from build123d import *

# Parameters (mm, degrees)
BOSS_EXTRU_1_DEPTH = 5
CONG_1_R           = 3


with BuildPart() as part:
    # Esquisse1 → Boss.-Extru.1 (new body)
    with BuildSketch(Plane.XY):
        with BuildLine():
            Line((0, -5), (0, 0))
            Line((0, 0), (-15, 0))
            Line((-15, 0), (-21.92820323, -9.797958971))
            Line((-21.92820323, -9.797958971), (-26.010686135, -6.911207626))
            Line((-26.010686135, -6.911207626), (-28.89743748, -10.99369053))
            Line((-28.89743748, -10.99369053), (-24.814954576, -13.880441876))
            Line((-24.814954576, -13.880441876), (-26.835680518, -16.73817991))
            Line((-26.835680518, -16.73817991), (-24.386190775, -18.470230717))
            Line((-24.386190775, -18.470230717), (-23.751105479, -17.572084478))
            Line((-23.751105479, -17.572084478), (-21.873163342, -18.899990097))
            Line((-21.873163342, -18.899990097), (-22.508248639, -19.798136336))
            Line((-22.508248639, -19.798136336), (-18.670714708, -22.511682601))
            Line((-18.670714708, -22.511682601), (-20.402765515, -24.961172344))
            Line((-20.402765515, -24.961172344), (-24.240299446, -22.247626079))
            Line((-24.240299446, -22.247626079), (-24.875384742, -23.145772318))
            Line((-24.875384742, -23.145772318), (-26.753326878, -21.817866699))
            Line((-26.753326878, -21.817866699), (-26.118241582, -20.91972046))
            Line((-26.118241582, -20.91972046), (-28.567731325, -19.187669652))
            Line((-28.567731325, -19.187669652), (-30.588457267, -22.045407686))
            Line((-30.588457267, -22.045407686), (-34.670940172, -19.15865634))
            Line((-34.670940172, -19.15865634), (-37.557691518, -23.241139245))
            Line((-37.557691518, -23.241139245), (-33.475208613, -26.127890591))
            Line((-33.475208613, -26.127890591), (-36.361959959, -30.210373495))
            Line((-36.361959959, -30.210373495), (-40.444442863, -27.32362215))
            Line((-40.444442863, -27.32362215), (-43.331194209, -31.406105054))
            Line((-43.331194209, -31.406105054), (-39.248711304, -34.2928564))
            Line((-39.248711304, -34.2928564), (-41.269437246, -37.150594433))
            Line((-41.269437246, -37.150594433), (-38.819947503, -38.882645241))
            Line((-38.819947503, -38.882645241), (-38.184862207, -37.984499002))
            Line((-38.184862207, -37.984499002), (-36.306920071, -39.312404621))
            Line((-36.306920071, -39.312404621), (-36.942005367, -40.21055086))
            Line((-36.942005367, -40.21055086), (-33.104471437, -42.924097125))
            Line((-33.104471437, -42.924097125), (-34.836522244, -45.373586868))
            Line((-34.836522244, -45.373586868), (-38.674056175, -42.660040603))
            Line((-38.674056175, -42.660040603), (-39.309141471, -43.558186842))
            Line((-39.309141471, -43.558186842), (-41.187083607, -42.230281223))
            Line((-41.187083607, -42.230281223), (-40.551998311, -41.332134984))
            Line((-40.551998311, -41.332134984), (-43.001488054, -39.600084176))
            Line((-43.001488054, -39.600084176), (-45.022213996, -42.45782221))
            Line((-45.022213996, -42.45782221), (-49.104696901, -39.571070864))
            Line((-49.104696901, -39.571070864), (-51.991448246, -43.653553769))
            Line((-51.991448246, -43.653553769), (-47.908965342, -46.540305114))
            Line((-47.908965342, -46.540305114), (-50.795716687, -50.622788019))
            ThreePointArc((-50.795716687, -50.622788019), (-33.780137683, -59.08727806), (-15, -62))
            Line((-15, -62), (0, -62))
            Line((0, -62), (0, -57))
            Line((0, -57), (5, -57))
            Line((5, -57), (5, -52))
            Line((5, -52), (0, -52))
            Line((0, -52), (0, -48.5))
            Line((0, -48.5), (-3, -48.5))
            Line((-3, -48.5), (-3, -49.6))
            Line((-3, -49.6), (-5.3, -49.6))
            Line((-5.3, -49.6), (-5.3, -48.5))
            Line((-5.3, -48.5), (-10, -48.5))
            Line((-10, -48.5), (-10, -45.5))
            Line((-10, -45.5), (-5.3, -45.5))
            Line((-5.3, -45.5), (-5.3, -44.4))
            Line((-5.3, -44.4), (-3, -44.4))
            Line((-3, -44.4), (-3, -45.5))
            Line((-3, -45.5), (0, -45.5))
            Line((0, -45.5), (0, -42))
            Line((0, -42), (5, -42))
            Line((5, -42), (5, -37))
            Line((5, -37), (0, -37))
            Line((0, -37), (0, -25))
            Line((0, -25), (5, -25))
            Line((5, -25), (5, -20))
            Line((5, -20), (0, -20))
            Line((0, -20), (0, -16.5))
            Line((0, -16.5), (-3, -16.5))
            Line((-3, -16.5), (-3, -17.6))
            Line((-3, -17.6), (-5.3, -17.6))
            Line((-5.3, -17.6), (-5.3, -16.5))
            Line((-5.3, -16.5), (-10, -16.5))
            Line((-10, -16.5), (-10, -13.5))
            Line((-10, -13.5), (-5.3, -13.5))
            Line((-5.3, -13.5), (-5.3, -12.4))
            Line((-5.3, -12.4), (-3, -12.4))
            Line((-3, -12.4), (-3, -13.5))
            Line((-3, -13.5), (0, -13.5))
            Line((0, -13.5), (0, -10))
            Line((0, -10), (5, -10))
            Line((5, -10), (5, -5))
            Line((5, -5), (0, -5))
        make_face()
    extrude(amount=BOSS_EXTRU_1_DEPTH)

    # Congé1
    cong_1_edges = [part.edges().sort_by_distance(p)[0] for p in [
        (-15, 0, 2.5),
    ]]
    fillet(cong_1_edges, radius=CONG_1_R)


solid = part.part
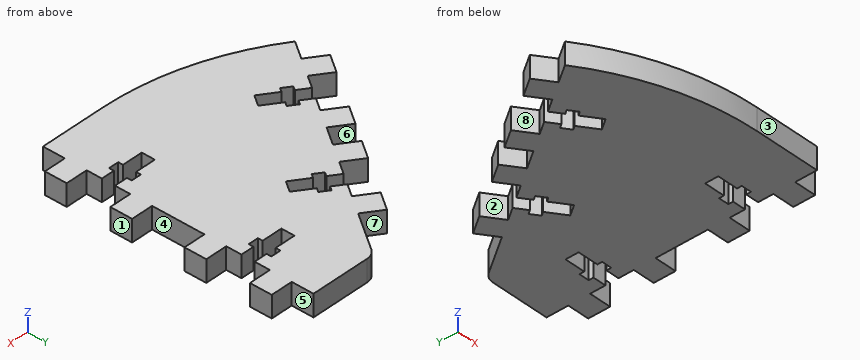
Verification items for the finished model (mm, model axes). Face numbers are marked on the shaded views. A direction names the side the tool comes from. Give positions to 0.01 mm unless a question says otherwise; leave off trailing zeros. Write each loop counter-clockwise with the first axis right and the second up, starting at its lowest first coordinate (ties: lowest second). Pieces come first, ordered by that corner, then holes. Notation, with made-up numbers: M 21,35.5 L 59,35.5 A12 cw 59,44.5 Z; hole C 11.5,36.25 d11. An arc over 180 degrees is marked long. Use CSV: the item, a comma, the result in double quotes.
1) Material ranges on line 1 along Y through (x, z) = (-1.5, 3.2); line 2 along Y through (x, z) = (-22, 4.65); line 3 along Y through (x, z) = (-39, 2.7) (3 decimals), recorded low to high.
Final values:
line 1,"-62 to -48.5, -45.5 to -16.5, -13.5 to 0"
line 2,"-61.6 to -23.83, -20.16 to -19.08, -18.81 to -9.75"
line 3,"-57.166 to -43.121, -38.755 to -28.345"
2) Go/stop test with flat-tipped pins: pin 1 Ø3 at (y, z) = (-20.5, 3.5) entering from -X; pin 2 Ø2.5 at (x, z) = (3.5, 2.5) entering from +Y; pin 3 Ø0.9 at (y, z) = (-45, 3.5) entering from +X. Record where each tip stops, or that it passes through.
Final values:
pin 1,"x = -36.68"
pin 2,"y = -5"
pin 3,"x = 0"
3) Cross-section at B-B (x = -7). Enter the section's corners in (y, z), plus the area to 3 significant figures.
Final values:
outline,"M -62,0 L -48.5,0 L -48.5,5 L -62,5 Z; M -45.5,0 L -16.5,0 L -16.5,5 L -45.5,5 Z; M -13.5,0 L 0,0 L 0,5 L -13.5,5 Z"
area,"280 mm²"
4) Release check for a two-part mould opening along Y. For the marked faces 1, 2 and 3 record: released by +Y, released by -Y, zero draft, split by the parting line, or undercut.
Final values:
face 1,"zero draft"
face 2,"undercut"
face 3,"released by -Y"
5) Access from +Z, -Z, +X, -X, +Y, -Y to the whole of each face (thin tool, end or side, straight path). Record for the marked faces 4, 5, 6, 7 and 8.
Final values:
face 4,"+Z, -Z, +X"
face 5,"+Z, -Z, +X, +Y"
face 6,"+Z, -Z"
face 7,"+Z, -Z, +Y"
face 8,"+Z, -Z, -X"
6) Cross-section at A-A (x = 1). Enter the section's corners in (y, z).
Final values:
outline,"M -57,0 L -52,0 L -52,5 L -57,5 Z; M -42,0 L -37,0 L -37,5 L -42,5 Z; M -25,0 L -20,0 L -20,5 L -25,5 Z; M -10,0 L -5,0 L -5,5 L -10,5 Z"
7) Cross-section at C-C (y = -15). Enter the section's corners in (x, z), plus the area to 3 significant figures.
Final values:
outline,"M -25.61,0 L -10,0 L -10,5 L -25.61,5 Z"
area,"78.0 mm²"
